Source: CAD feature listing. Evaluate the final solid. Frame: model axes, mm. A direction names the side the tool comes from. Round coordinates to 2 decimals unless told otherwise and drop trailing zeros. Write each loop counter-clockwise with the first axis right and the second up, starting at its lowest first coordinate (ties: lowest second). Pieces come first, ordered by that corner, then holes.
from build123d import *

# Parameters (mm, degrees)
SKETCH1_R           = 12
BOSS_EXTRUDE1_DEPTH = 10
BOSS_EXTRUDE2_DEPTH = 35
FILLET1_R           = 15


with BuildPart() as part:
    # Sketch1 → Boss-Extrude1 (new body)
    with BuildSketch(Plane(origin=(0, 0, 0), x_dir=(1, 0, 0), z_dir=(0, 1, 0))):
        Polygon((40, 25), (0, 25), (0, 15), (-30, 15), (-30, -15), (0, -15), (0, -25), (40, -25), align=None)
        with Locations(Location((15, 0, 0), (0, 0, 270))):
            Circle(SKETCH1_R, mode=Mode.SUBTRACT)
    extrude(amount=BOSS_EXTRUDE1_DEPTH)

    # Sketch1_3 → Boss-Extrude2 (add)
    with BuildSketch(Plane(origin=(0, 0, 0), x_dir=(1, 0, 0), z_dir=(0, 1, 0))):
        Polygon((0, 15), (0, 25), (-40, 25), (-40, -25), (0, -25), (0, -15), (-30, -15), (-30, 15), align=None)
    extrude(amount=BOSS_EXTRUDE2_DEPTH)

    # Fillet1
    fillet1_edges = [part.edges().sort_by_distance(p)[0] for p in [
        (40, 5, -25),
        (40, 5, 25),
    ]]
    fillet(fillet1_edges, radius=FILLET1_R)


solid = part.part
1) Section query A-A on z = 0. Return the cut outline in (x, y), then the cut area to 3 significant figures.
Taken from the geometry:
outline: (-40, 0) - (3, 0) - (3, 10) - (-30, 10) - (-30, 35) - (-40, 35) - close; (27, 0) - (40, 0) - (40, 10) - (27, 10) - close
area: 810 mm2
2) Section query B-B on y = 7. Return the cut outline in (x, z).
Taken from the geometry:
outline: (-40, -25) - (25, -25) arc R15 ccw to (40, -10) - (40, 10) arc R15 ccw to (25, 25) - (-40, 25) - close; hole circle Ø24 at (15, 0)
3) Material intervals for line 1 (X direction, y = 4, z = 0); line 2 (Z direction, x = -5.5, y = 17.5); line 3 (Y direction, x = -12.5, z = -12), sorted ascending.
Taken from the geometry:
line 1: x = -40 to 3, 27 to 40
line 2: z = -25 to -15, 15 to 25
line 3: y = 0 to 10
4) Section query C-C on y = 28. Return the cut outline in (x, z).
Taken from the geometry:
outline: (-40, -25) - (0, -25) - (0, -15) - (-30, -15) - (-30, 15) - (0, 15) - (0, 25) - (-40, 25) - close
5) Contact query for flat-ended pins moving along their axis: P1, Ø1, axis at x = 28.5, y = 12, coming from the +Z side; P2, Ø8, axis at y = 21.5, z = 20.5, coming from the +X side; P3, Ø5, axis at x = 9, z = -11.5, coming from the +Y side. Output: stop coordinate, or through.
Taken from the geometry:
P1: passes through
P2: stops at x = 0
P3: stops at y = 10
6) Section query D-D on x = 16. Return the cut outline in (y, z), then the cut area to 3 significant figures.
Taken from the geometry:
outline: (0, -25) - (10, -25) - (10, -11.96) - (0, -11.96) - close; (0, 11.96) - (10, 11.96) - (10, 25) - (0, 25) - close
area: 261 mm2
7) Pull-direction query (Z, two-part tool) for faces 1 (the face through (35.72, 5.07, -20.49)), 2 (the face through (-3, 10, 0)), 3 (the face through (-1, 0, 0)); classes: released by +Z, released by -Z, zero draft, split by the parting line, or undercut.
Taken from the geometry:
face 1: released by -Z
face 2: undercut
face 3: zero draft
8) Reachability of faces 4 (the face through (0, 22, 20)), 5 (the face through (18.604, 4.93, 11.446)), 6 (the face through (-15, 22, -15)) from +Z, -Z, +X, -X, +Y, -Y: full face, straight path, thin tool, end or side. Return the list, or none.
Taken from the geometry:
face 4: +Z, -Z, +X, +Y
face 5: +Y, -Y
face 6: +X, +Y
